from build123d import *
from OCP.BRepFilletAPI import BRepFilletAPI_MakeChamfer

# Parameters (mm, degrees)
BOSS_EXTRUDE2_DEPTH = 1
SKETCH4_R           = 0.8
CUT_EXTRUDE1_DEPTH  = 31.551677532
SKETCH5_W           = 9.1
SKETCH5_H           = 3.25
CUT_EXTRUDE2_DEPTH  = 31.551677532
FILLET1_R           = 1.3
CHAMFER1_SIZE       = 0.75
CHAMFER1_SIZE2      = 0.433012702


with BuildPart() as part:
    # Sketch3 → Boss-Extrude2 (new body)
    with BuildSketch(Plane.XY):
        with BuildLine():
            Line((24, 5.95), (-24, 5.95))
            ThreePointArc((-24, 5.95), (-29.95, 0), (-24, -5.95))
            Line((-24, -5.95), (24, -5.95))
            ThreePointArc((24, -5.95), (29.95, 0), (24, 5.95))
        make_face()
    extrude(amount=BOSS_EXTRUDE2_DEPTH)

    # Sketch4 → Cut-Extrude1 (cut, through all)
    with BuildSketch(Plane.XY.offset(1)):
        with Locations((-27, 0)):
            Circle(SKETCH4_R)
        with Locations((27, 0)):
            Circle(SKETCH4_R)
    extrude(amount=-CUT_EXTRUDE1_DEPTH, mode=Mode.SUBTRACT)

    # Sketch5 → Cut-Extrude2 (cut, through all)
    with BuildSketch(Plane(origin=(0, 0, 0), x_dir=(-1, 0, 0), z_dir=(0, 0, -1))):
        with Locations((0.5, -0.725)):
            Rectangle(SKETCH5_W, SKETCH5_H)
    extrude(amount=-CUT_EXTRUDE2_DEPTH, mode=Mode.SUBTRACT)

    # Fillet1
    fillet1_edges = [part.edges().sort_by_distance(p)[0] for p in [
        (4.05, -2.35, 0.5),
        (4.05, 0.9, 0.5),
        (-5.05, 0.9, 0.5),
        (-5.05, -2.35, 0.5),
    ]]
    fillet(fillet1_edges, radius=FILLET1_R)

    # Chamfer1: one chamfer whose edges measure the first distance from different faces: ONE call of the kernel's chamfer builder (chamfer() names one face for all edges)
    chamfer1_edges_1 = [part.edges().sort_by_distance(p)[0] for p in [
        (-27.8, 0, 0),
    ]]
    chamfer1_side_1 = [part.faces().sort_by_distance(p)[0] for p in [
        (-27.8, 0, 0.5),
    ]]
    chamfer1_edges_2 = [part.edges().sort_by_distance(p)[0] for p in [
        (26.2, 0, 0),
    ]]
    chamfer1_side_2 = [part.faces().sort_by_distance(p)[0] for p in [
        (26.2, 0, 0.5),
    ]]
    chamfer1 = BRepFilletAPI_MakeChamfer(part.part.solid().wrapped)
    for e in chamfer1_edges_1:
        chamfer1.Add(CHAMFER1_SIZE, CHAMFER1_SIZE2, e.wrapped, chamfer1_side_1[0].wrapped)  # the first distance lies on this face
    for e in chamfer1_edges_2:
        chamfer1.Add(CHAMFER1_SIZE, CHAMFER1_SIZE2, e.wrapped, chamfer1_side_2[0].wrapped)  # the first distance lies on this face
    add(Compound.cast(chamfer1.Shape()), mode=Mode.REPLACE)


solid = part.part
Design review of the part built by this model. Coordinates are the model's own, in mm. A direction names the side the tool comes from. Coordinates: 2 decimals unless noted, no trailing zeros. Order: outer loops, then holes, each group sorted by start corner. A loop starts at its lowest first (then second) coordinate and runs counter-clockwise, first axis right, second up. Notation, with made-up numbers: (8.5, 4) -> (13.5, 4) arc R8 ccw to (13.5, 8) -> close; hole circle Ø4 at (-6.75, 72.25). An arc over 180 degrees is marked (long way). Use one line per item in the form item = value. Start each with the question number.
(1) Add section D-D on x = 27. State the section outline as (y, z) points.
(2) Add section C-C on y = 2.5. State the section outline as (x, z) points, plus the area to 3 significant figures.
(3) For probe 1 along Y at (x, z) = (1.5, 0.8); probe 2 along Y at (x, z) = (-27, 0.9); probe 3 along X at (y, z) = (-1.5, 0.65), list the stretches that pass through material, from the lowest coordinate up.
(4) The part is to be moulded in two halves that separate along X. For faces 3 (the cylindrical face through (-4.68, -1.96, 0.51)), 4 (the cylindrical face through (29.95, -0.13, 0.49)), 5 (the flat face through (-0.5, -2.35, 0.5)), 6 (the cylindrical face through (-29.95, 0.13, 0.49)), say which applies: +X half, -X half, draft (parallel to the pull), parting line (faces both ways), or undercut.
(5) Insertion check: pin 1 (0.5 mm diameter, centred on y = -0.5, z = 0.5, fed in from +X); pin 2 (1 mm diameter, centred on x = 27, y = 0, fed in from +Z). Each pin has a flat end and moves straight along its axis. Give the tip position at first contact, or say it passes through.
(6) Add section A-A on x = 3.5. State the section outline as (y, z) points, plus the area to 3 significant figures.
(7) Add section B-B on z = 0.55. State the section outline as (x, y) points.
(8) For faces 1 (the flat face through (-0.4, 1.4, 0)), 2 (the flat face through (-0.5, 0.9, 0.5)), list the 3-axis set-ups (+Z, -Z, +X, -X, +Y, -Y) from which the entire face can be reached by the end or side of a thin tool; tool diameter is ignored.
Answer block:
q1.outline = (-5.14, 0) -> (-1.23, 0) -> (-0.8, 0.75) -> (-0.8, 1) -> (-5.14, 1) -> close; (0.8, 0.75) -> (1.23, 0) -> (5.14, 0) -> (5.14, 1) -> (0.8, 1) -> close
q2.outline = (-29.4, 0) -> (29.4, 0) -> (29.4, 1) -> (-29.4, 1) -> close
q2.area = 58.8 mm²
q3.probe_1 = -5.95 to -2.35, 0.9 to 5.95
q3.probe_2 = -5.14 to -0.8, 0.8 to 5.14
q3.probe_3 = -29.76 to -4.97, 3.97 to 29.76
q4.face_3 = undercut
q4.face_4 = +X half
q4.face_5 = undercut
q4.face_6 = -X half
q5.pin_1 = 29.94
q5.pin_2 = through
q6.outline = (-5.95, 0) -> (-2.11, 0) -> (-2.11, 1) -> (-5.95, 1) -> close; (0.66, 0) -> (5.95, 0) -> (5.95, 1) -> (0.66, 1) -> close
q6.area = 9.13 mm²
q7.outline = (-24, -5.95) -> (24, -5.95) arc R5.95 ccw to (24, 5.95) -> (-24, 5.95) arc R5.95 ccw to start; hole circle Ø1.83 at (-27, 0); hole (-5.05, -1.05) arc R1.3 ccw to (-3.75, -2.35) -> (2.75, -2.35) arc R1.3 ccw to (4.05, -1.05) -> (4.05, -0.4) arc R1.3 ccw to (2.75, 0.9) -> (-3.75, 0.9) arc R1.3 ccw to (-5.05, -0.4) -> close; hole circle Ø1.83 at (27, 0)
q8.face_1 = -Z, +X, -X, +Y, -Y
q8.face_2 = +Z, -Z
